Read the model definition and answer for the solid it produces. Units are mm, in the model's axes. Face numbers are marked on the shaded views. Coordinates: 2 decimals unless noted, no trailing zeros. Order: outer loops, then holes, each group sorted by start corner. A loop starts at its lowest first (then second) coordinate and runs counter-clockwise, first axis right, second up. Notation, with made-up numbers: M 45,33.5 L 67,33.5 A30 cw 67,62.5 Z; hole C 55.5,1 d8. An arc over 180 degrees is marked long. One line per question, with ' | ' between items. Start each with the question number.
1) Find section D-D, the plane y = -41. Write down the section's boundary in (x, z).
2) Find section B-B, the plane y = -4. Write down the section's boundary in (x, z), plus the area to 3 significant figures.
3) Find section C-C, the plane x = 37.5. Write down the section's boundary in (y, z), plus the area to 3 significant figures.
4) Consider probe 1 along X at (y, z) = (-23.5, 2); probe 2 along Z at (x, y) = (17, -19); probe 3 along Y at (x, z) = (38.5, 16). Determine where each line is inside the solid, lowest interval first.
5) Find section A-A, the plane z = 27.5. Write down the section's boundary in (x, y), plus the area to 3 significant figures.
6) Given P1, Ø8, axis at y = -20, z = 8, coming from the -X side; P2, Ø3, axis at y = -13, z = 27.5, coming from the -X side; P3, Ø4, axis at y = -31.5, z = 19.5, coming from the -X side, each flat-ended and moving along its own axis, determine where each tip first touches the part or whether it passes through.
7) The mould has two halves that part along X. Classify the marked faces 1, 2 and 3: +X half, -X half, draft (parallel to the pull), parting line (faces both ways), or undercut.
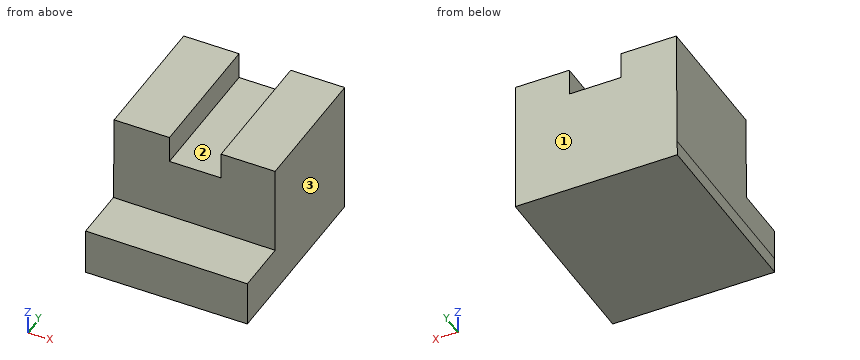
from build123d import *

# Parameters (mm, degrees)
F1_DEPTH = 19.05
F2_DEPTH = 25.4
F3_DEPTH = 25.4
F5_DEPTH = 12.7


with BuildPart() as f1:
    # F0 (on Front) → F1 (new body)
    with BuildSketch(Plane.XZ):
        Polygon((2.828845887, 3.5896749168), (2.8014711667, 0), (40.9014711667, 0), (40.9014711667, 3.2993345685), align=None)
        Polygon((2.9930308781, 25.1194198566), (2.828845887, 3.5896749168), (40.9014711667, 3.2993345685), (40.9014711667, 25.3031502977), (28.2014711667, 25.4), (16.0545626627, 25.4), align=None)
        Polygon((3.0435954224, 31.75), (2.9930308781, 25.1194198566), (16.0545626627, 25.4), (16.0545626627, 31.75), align=None)
        Polygon((28.2014711667, 25.4), (40.9014711667, 25.3031502977), (40.9014711667, 31.75), (28.2014711667, 31.75), align=None)
    extrude(amount=F1_DEPTH)

    # F0 (on Front) → F2 (cut)
    with BuildSketch(Plane.XZ):
        Polygon((2.828845887, 3.5896749168), (2.8014711667, 0), (40.9014711667, 0), (40.9014711667, 3.2993345685), align=None)
        Polygon((2.9930308781, 25.1194198566), (2.828845887, 3.5896749168), (40.9014711667, 3.2993345685), (40.9014711667, 25.3031502977), (28.2014711667, 25.4), (16.0545626627, 25.4), align=None)
        Polygon((3.0435954224, 31.75), (2.9930308781, 25.1194198566), (16.0545626627, 25.4), (16.0545626627, 31.75), align=None)
        Polygon((28.2014711667, 25.4), (40.9014711667, 25.3031502977), (40.9014711667, 31.75), (28.2014711667, 31.75), align=None)
    extrude(amount=-F2_DEPTH, mode=Mode.SUBTRACT)

    # F3 (add): a face of the model
    f3_faces = [f1.faces().sort_by_distance(p)[0] for p in [
        (21.8971715309, -19.05, 14.989088292),
    ]]
    extrude(f3_faces, amount=F3_DEPTH)

    # F4 (on face) → F5 (cut)
    with BuildSketch(Plane.XZ.offset(44.45)):
        Polygon((3.0435954224, 31.75), (2.8853301618, 10.9965153512), (40.9014711667, 10.7066057497), (40.9014711667, 31.75), (28.2014711667, 31.75), (28.2014711667, 25.4), (16.0545626627, 25.4), (16.0545626627, 31.75), align=None)
    extrude(amount=-F5_DEPTH, mode=Mode.SUBTRACT)


solid = f1.part
Report:
1) outline: M 2.8,0 L 40.9,0 L 40.9,10.71 L 2.89,11 Z
2) outline: M 2.8,0 L 40.9,0 L 40.9,31.75 L 28.2,31.75 L 28.2,25.4 L 16.05,25.4 L 16.05,31.75 L 3.04,31.75 Z | area: 1,130 mm^2
3) outline: M -44.45,0 L 0,0 L 0,31.75 L -31.75,31.75 L -31.75,10.73 L -44.45,10.73 Z | area: 1,140 mm^2
4) probe 1: x = 2.82 to 40.9 | probe 2: z = 0 to 25.4 | probe 3: y = -31.75 to 0
5) outline: M 3.01,-31.75 L 16.05,-31.75 L 16.05,0 L 3.01,0 Z; M 28.2,-31.75 L 40.9,-31.75 L 40.9,0 L 28.2,0 Z | area: 817 mm^2
6) P1: stops at x = 2.83 | P2: stops at x = 3 | P3: stops at x = 2.93
7) face 1: draft | face 2: undercut | face 3: +X half
